Geometry: final body of the model. Coordinates: model frame, mm. A direction names the side the tool comes from. Coordinates: 2 decimals unless noted, no trailing zeros. Order: outer loops, then holes, each group sorted by start corner. A loop starts at its lowest first (then second) coordinate and runs counter-clockwise, first axis right, second up. Notation, with made-up numbers: (-8, -26.75) -> (-2, -26.75) arc R18 ccw to (-2, -15.75) -> close; hole circle Ø9 at (34, -12.5). An arc over 180 degrees is marked (long way). Use one line per item in the form item = value.
```python
from build123d import *

# Parameters (mm, degrees)
SKETCH1_W           = 96
SKETCH1_H           = 28
BOSS_EXTRUDE1_DEPTH = 3
SKETCH2_W           = 3
SKETCH2_H           = 25
BOSS_EXTRUDE2_DEPTH = 25
SKETCH3_W           = 96
SKETCH3_H           = 35
BOSS_EXTRUDE3_DEPTH = 3
CUT_EXTRUDE2_REACH  = 30
SKETCH4_R           = 1.5
SKETCH5_R           = 3.5
CUT_EXTRUDE3_DEPTH  = 0.7
CUT_EXTRUDE4_REACH  = 33
SKETCH6_R           = 1.5
SKETCH6_R_2         = 1.25
SKETCH7_R           = 4
CUT_EXTRUDE5_DEPTH  = 2
CUT_EXTRUDE7_REACH  = 33
SKETCH8_R           = 3
SKETCH8_W           = 25
SKETCH8_H           = 12
CUT_EXTRUDE8_REACH  = 5
SKETCH9_W           = 20
SKETCH9_H           = 10
SKETCH9_W_2         = 9
CUT_EXTRUDE9_REACH  = 5
SKETCH10_W          = 25
SKETCH10_H          = 8


with BuildPart() as part:
    # Sketch1 → Boss-Extrude1 (new body)
    with BuildSketch(Plane(origin=(0, 0, 0), x_dir=(1, 0, 0), z_dir=(0, 1, 0))):
        with Locations((2.671135036, -161.861135542)):
            Rectangle(SKETCH1_W, SKETCH1_H)
    extrude(amount=BOSS_EXTRUDE1_DEPTH)

    # Sketch2 → Boss-Extrude2 (add)
    with BuildSketch(Plane(origin=(0, 0, 0), x_dir=(-1, 0, 0), z_dir=(0, -1, 0))):
        Polygon((-50.671135036, -175.861135542), (45.328864964, -175.861135542), (45.328864964, -172.861135542), (42.328864964, -172.861135542), (-47.671135036, -172.861135542), (-50.671135036, -172.861135542), align=None)
        with Locations((43.828864964, -160.361135542)):
            Rectangle(SKETCH2_W, SKETCH2_H)
        with Locations((-49.171135036, -160.361135542)):
            Rectangle(SKETCH2_W, SKETCH2_H)
    extrude(amount=BOSS_EXTRUDE2_DEPTH)

    # Sketch3 → Boss-Extrude3 (add)
    with BuildSketch(Plane(origin=(0, 0, 147.861135542), x_dir=(-1, 0, 0), z_dir=(0, 0, -1))):
        with Locations((-2.671135036, -7.5)):
            Rectangle(SKETCH3_W, SKETCH3_H)
    extrude(amount=BOSS_EXTRUDE3_DEPTH)

    # Sketch4 → Cut-Extrude2 (cut, up to next)
    with BuildSketch(Plane(origin=(0, 3, 0), x_dir=(1, 0, 0), z_dir=(0, 1, 0)), mode=Mode.PRIVATE) as cut_extrude2_sk1:
        with Locations((-19.828864964, -160.361135542)):
            Circle(SKETCH4_R)
    cut_extrude2_tool1 = extrude(cut_extrude2_sk1.sketch, amount=-CUT_EXTRUDE2_REACH, mode=Mode.PRIVATE) & part.part
    add(cut_extrude2_tool1.solids().sort_by_distance((-19.828865, 3, 160.361136))[0], mode=Mode.SUBTRACT)
    # Sketch4 → Cut-Extrude2 (cut, up to next)
    with BuildSketch(Plane(origin=(0, 3, 0), x_dir=(1, 0, 0), z_dir=(0, 1, 0)), mode=Mode.PRIVATE) as cut_extrude2_sk2:
        with Locations((25.171135036, -160.361135542)):
            Circle(SKETCH4_R)
    cut_extrude2_tool2 = extrude(cut_extrude2_sk2.sketch, amount=-CUT_EXTRUDE2_REACH, mode=Mode.PRIVATE) & part.part
    add(cut_extrude2_tool2.solids().sort_by_distance((25.171135, 3, 160.361136))[0], mode=Mode.SUBTRACT)

    # Sketch5 → Cut-Extrude3 (cut)
    with BuildSketch(Plane(origin=(0, 3, 0), x_dir=(1, 0, 0), z_dir=(0, 1, 0))):
        with Locations((-19.828864964, -160.361135542)):
            Circle(SKETCH5_R)
        with Locations((25.171135036, -160.361135542)):
            Circle(SKETCH5_R)
    extrude(amount=-CUT_EXTRUDE3_DEPTH, mode=Mode.SUBTRACT)

    # Sketch6 → Cut-Extrude4 (cut, up to next)
    with BuildSketch(Plane(origin=(0, 0, 144.861135542), x_dir=(-1, 0, 0), z_dir=(0, 0, -1)), mode=Mode.PRIVATE) as cut_extrude4_sk1:
        with Locations((-18.921135036, -2)):
            Circle(SKETCH6_R)
    cut_extrude4_tool1 = extrude(cut_extrude4_sk1.sketch, amount=-CUT_EXTRUDE4_REACH, mode=Mode.PRIVATE) & part.part
    add(cut_extrude4_tool1.solids().sort_by_distance((18.921135, -2, 144.861136))[0], mode=Mode.SUBTRACT)
    # Sketch6 → Cut-Extrude4 (cut, up to next)
    with BuildSketch(Plane(origin=(0, 0, 144.861135542), x_dir=(-1, 0, 0), z_dir=(0, 0, -1)), mode=Mode.PRIVATE) as cut_extrude4_sk2:
        with Locations((13.578864964, -2)):
            Circle(SKETCH6_R)
    cut_extrude4_tool2 = extrude(cut_extrude4_sk2.sketch, amount=-CUT_EXTRUDE4_REACH, mode=Mode.PRIVATE) & part.part
    add(cut_extrude4_tool2.solids().sort_by_distance((-13.578865, -2, 144.861136))[0], mode=Mode.SUBTRACT)
    # Sketch6 → Cut-Extrude4 (cut, up to next)
    with BuildSketch(Plane(origin=(0, 0, 144.861135542), x_dir=(-1, 0, 0), z_dir=(0, 0, -1)), mode=Mode.PRIVATE) as cut_extrude4_sk3:
        with Locations((12.328864964, 7.5)):
            Circle(SKETCH6_R_2)
    cut_extrude4_tool3 = extrude(cut_extrude4_sk3.sketch, amount=-CUT_EXTRUDE4_REACH, mode=Mode.PRIVATE) & part.part
    add(cut_extrude4_tool3.solids().sort_by_distance((-12.328865, 7.5, 144.861136))[0], mode=Mode.SUBTRACT)
    # Sketch6 → Cut-Extrude4 (cut, up to next)
    with BuildSketch(Plane(origin=(0, 0, 144.861135542), x_dir=(-1, 0, 0), z_dir=(0, 0, -1)), mode=Mode.PRIVATE) as cut_extrude4_sk4:
        with Locations((-17.671135036, 7.5)):
            Circle(SKETCH6_R_2)
    cut_extrude4_tool4 = extrude(cut_extrude4_sk4.sketch, amount=-CUT_EXTRUDE4_REACH, mode=Mode.PRIVATE) & part.part
    add(cut_extrude4_tool4.solids().sort_by_distance((17.671135, 7.5, 144.861136))[0], mode=Mode.SUBTRACT)

    # Sketch7 → Cut-Extrude5 (cut)
    with BuildSketch(Plane.XY.offset(147.861135542)):
        with Locations((18.921135036, -2)):
            Circle(SKETCH7_R)
        with Locations((-13.578864964, -2)):
            Circle(SKETCH7_R)
    extrude(amount=-CUT_EXTRUDE5_DEPTH, mode=Mode.SUBTRACT)

    # Sketch8 → Cut-Extrude7 (cut, up to next)
    with BuildSketch(Plane.XY.offset(175.861135542), mode=Mode.PRIVATE) as cut_extrude7_sk1:
        with Locations((2.671135036, -10)):
            Circle(SKETCH8_R)
    cut_extrude7_tool1 = extrude(cut_extrude7_sk1.sketch, amount=-CUT_EXTRUDE7_REACH, mode=Mode.PRIVATE) & part.part
    add(cut_extrude7_tool1.solids().sort_by_distance((2.671135, -10, 175.861136))[0], mode=Mode.SUBTRACT)
    # Sketch8 → Cut-Extrude7 (cut, up to next)
    with BuildSketch(Plane.XY.offset(175.861135542), mode=Mode.PRIVATE) as cut_extrude7_sk2:
        with Locations((-14.828864964, -10)):
            Rectangle(SKETCH8_W, SKETCH8_H)
    cut_extrude7_tool2 = extrude(cut_extrude7_sk2.sketch, amount=-CUT_EXTRUDE7_REACH, mode=Mode.PRIVATE) & part.part
    add(cut_extrude7_tool2.solids().sort_by_distance((-14.828865, -10, 175.861136))[0], mode=Mode.SUBTRACT)
    # Sketch8 → Cut-Extrude7 (cut, up to next)
    with BuildSketch(Plane.XY.offset(175.861135542), mode=Mode.PRIVATE) as cut_extrude7_sk3:
        with Locations((20.171135036, -10)):
            Rectangle(SKETCH8_W, SKETCH8_H)
    cut_extrude7_tool3 = extrude(cut_extrude7_sk3.sketch, amount=-CUT_EXTRUDE7_REACH, mode=Mode.PRIVATE) & part.part
    add(cut_extrude7_tool3.solids().sort_by_distance((20.171135, -10, 175.861136))[0], mode=Mode.SUBTRACT)

    # Sketch9 → Cut-Extrude8 (cut, up to next)
    with BuildSketch(Plane.XY.offset(147.861135542), mode=Mode.PRIVATE) as cut_extrude8_sk1:
        with Locations((2.671135036, -12)):
            Rectangle(SKETCH9_W, SKETCH9_H)
    cut_extrude8_tool1 = extrude(cut_extrude8_sk1.sketch, amount=-CUT_EXTRUDE8_REACH, mode=Mode.PRIVATE) & part.part
    add(cut_extrude8_tool1.solids().sort_by_distance((2.671135, -12, 147.861136))[0], mode=Mode.SUBTRACT)
    # Sketch9 → Cut-Extrude8 (cut, up to next)
    with BuildSketch(Plane.XY.offset(147.861135542), mode=Mode.PRIVATE) as cut_extrude8_sk2:
        with Locations((-23.828864964, -12)):
            Rectangle(SKETCH9_W_2, SKETCH9_H)
    cut_extrude8_tool2 = extrude(cut_extrude8_sk2.sketch, amount=-CUT_EXTRUDE8_REACH, mode=Mode.PRIVATE) & part.part
    add(cut_extrude8_tool2.solids().sort_by_distance((-23.828865, -12, 147.861136))[0], mode=Mode.SUBTRACT)
    # Sketch9 → Cut-Extrude8 (cut, up to next)
    with BuildSketch(Plane.XY.offset(147.861135542), mode=Mode.PRIVATE) as cut_extrude8_sk3:
        with Locations((29.171135036, -12)):
            Rectangle(SKETCH9_W_2, SKETCH9_H)
    cut_extrude8_tool3 = extrude(cut_extrude8_sk3.sketch, amount=-CUT_EXTRUDE8_REACH, mode=Mode.PRIVATE) & part.part
    add(cut_extrude8_tool3.solids().sort_by_distance((29.171135, -12, 147.861136))[0], mode=Mode.SUBTRACT)

    # Sketch10 → Cut-Extrude9 (cut, up to next)
    with BuildSketch(Plane.ZY.offset(-47.671135036), mode=Mode.PRIVATE) as cut_extrude9_sk1:
        with Locations((160.361135542, -4)):
            Rectangle(SKETCH10_W, SKETCH10_H)
    cut_extrude9_tool1 = extrude(cut_extrude9_sk1.sketch, amount=-CUT_EXTRUDE9_REACH, mode=Mode.PRIVATE) & part.part
    add(cut_extrude9_tool1.solids().sort_by_distance((47.671135, -4, 160.361136))[0], mode=Mode.SUBTRACT)


solid = part.part
```
1) Pull-direction query (Y, two-part tool) for faces 5 (the flat face through (50.671, -12, 161)), 6 (the flat face through (12.671, -12, 146)), 7 (the flat face through (3, 10, 146)); classes: released by +Y, released by -Y, zero draft, split by the parting line, or undercut.
Results found:
face_5 = zero draft
face_6 = undercut
face_7 = released by +Y
2) Access query for faces 1 (the flat face through (32.671, -10, 174)), 2 (the flat face through (19, 1, 147.861)), 3 (the cylindrical face through (24.72, 2.65, 156.89)), 4 (the cylindrical face through (-12.08, -1.93, 145.35)). Directions: +Z, -Z, +X, -X, +Y, -Y. A direction counts if a zero-diameter tool reaches every point of the face in a straight line with its end or side. Return the directions, or none.
Results found:
face_1 = +Z
face_2 = none
face_3 = +Y
face_4 = -Z
3) Section C-C, the plane x = 9.5. Output: boundary loops of the cut face in (y, z).
Results found:
outline = (-25, 144.86) -> (-17, 144.86) -> (-17, 147.86) -> (-25, 147.86) -> close; (-25, 172.86) -> (-16, 172.86) -> (-16, 175.86) -> (-25, 175.86) -> close; (-7, 144.86) -> (10, 144.86) -> (10, 147.86) -> (3, 147.86) -> (3, 175.86) -> (-4, 175.86) -> (-4, 172.86) -> (0, 172.86) -> (0, 147.86) -> (-7, 147.86) -> close
4) Section B-B, the plane y = -15. Output: boundary loops of the cut face in (x, z).
Results found:
outline = (-45.33, 144.86) -> (-28.33, 144.86) -> (-28.33, 147.86) -> (-42.33, 147.86) -> (-42.33, 172.86) -> (-27.33, 172.86) -> (-27.33, 175.86) -> (-45.33, 175.86) -> close; (-19.33, 144.86) -> (-7.33, 144.86) -> (-7.33, 147.86) -> (-19.33, 147.86) -> close; (-2.33, 172.86) -> (7.67, 172.86) -> (7.67, 175.86) -> (-2.33, 175.86) -> close; (12.67, 144.86) -> (24.67, 144.86) -> (24.67, 147.86) -> (12.67, 147.86) -> close; (32.67, 172.86) -> (47.67, 172.86) -> (47.67, 147.86) -> (33.67, 147.86) -> (33.67, 144.86) -> (50.67, 144.86) -> (50.67, 175.86) -> (32.67, 175.86) -> close
5) Contact query for flat-ended pins moving along their axis: P1, Ø10, axis at x = -3.5, z = 153.5, coming from the +Y side; P2, Ø2.5, axis at x = 18.92, y = -2, coming from the -Z side; P3, Ø10.5, axis at x = -13.58, y = -2, coming from the -Z side; P4, Ø1, axis at x = 12, z = 165, coming from the -Y side. Output: stop coordinate, or through.
Results found:
P1 = 3
P2 = 172.86
P3 = 144.86
P4 = 0
6) Section A-A, the plane y = -2. Output: boundary loops of the cut face in (x, z), and give its area (3 significant figures).
Results found:
outline = (-45.33, 144.86) -> (-15.08, 144.86) -> (-15.08, 145.86) -> (-17.58, 145.86) -> (-17.58, 147.86) -> (-42.33, 147.86) -> (-42.33, 172.86) -> (50.67, 172.86) -> (50.67, 175.86) -> (-45.33, 175.86) -> close; (-12.08, 144.86) -> (17.42, 144.86) -> (17.42, 145.86) -> (14.92, 145.86) -> (14.92, 147.86) -> (-9.58, 147.86) -> (-9.58, 145.86) -> (-12.08, 145.86) -> close; (20.42, 144.86) -> (50.67, 144.86) -> (50.67, 147.86) -> (22.92, 147.86) -> (22.92, 145.86) -> (20.42, 145.86) -> close
area = 613 mm2
7) Material intervals for probe 1 along Y at (x, z) = (10, 146); probe 2 along X at (y, z) = (7, 146); probe 3 along Z at (x, y) = (44, -9.5), sorted ascending. Write a range as from..to.
Results found:
probe_1 = -25..-17, -7..10
probe_2 = -45.33..-13.47, -11.18..16.53, 18.82..50.67
probe_3 = 144.86..147.86, 172.86..175.86
8) Section D-D, the plane z = 169. Output: boundary loops of the cut face in (x, y).
Results found:
outline = (-45.33, -25) -> (-42.33, -25) -> (-42.33, 0) -> (50.67, 0) -> (50.67, 3) -> (-45.33, 3) -> close; (47.67, -25) -> (50.67, -25) -> (50.67, -8) -> (47.67, -8) -> close
